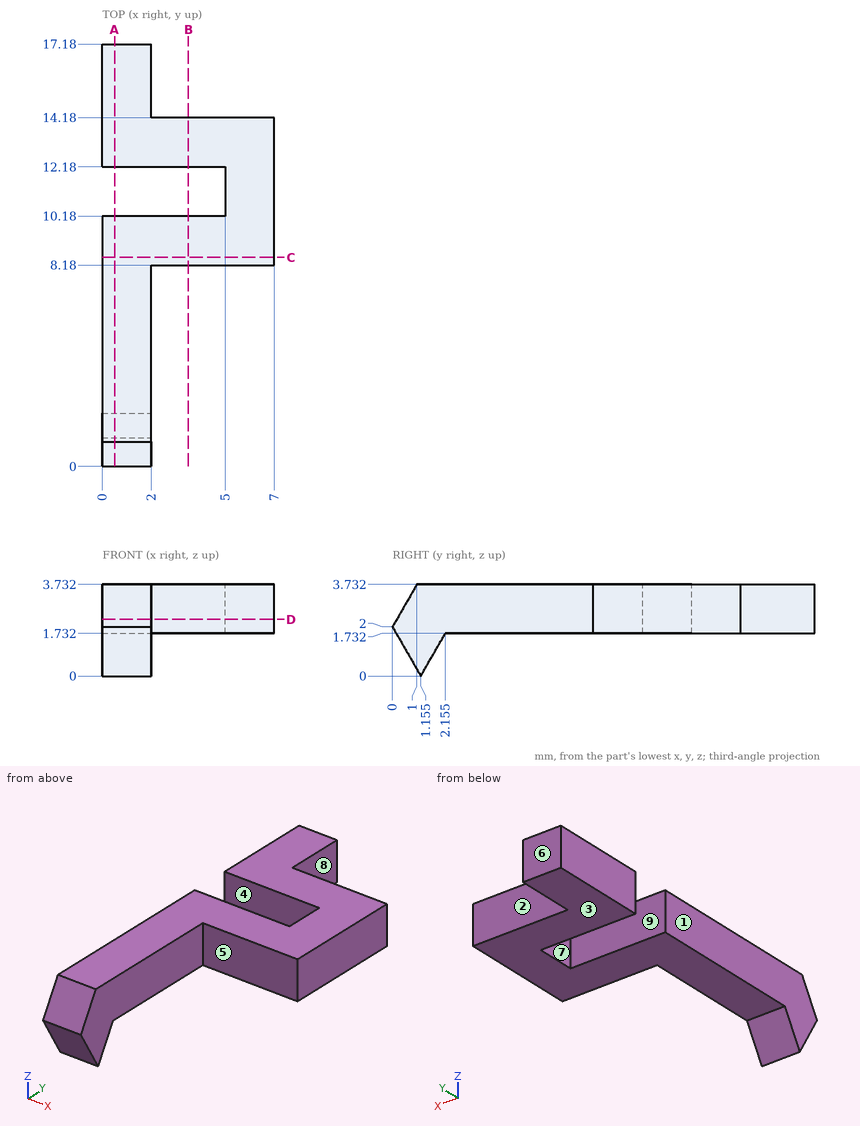
Geometry: see drawing. Coordinates: mm, zero at the bounding-box minimum. A direction names the side the tool comes from. Coordinates: 2 decimals unless noted, no trailing zeros. Order: outer loops, then holes, each group sorted by start corner. A loop starts at its lowest first (then second) coordinate and runs counter-clockwise, first axis right, second up. Notation, with made-up numbers: M -1,8 L 24,8 A22 ccw 24,16 Z; hole C 61.5,83.5 d4. An arc over 180 degrees is marked long. Write each question's results on one line, items separated by ' | '. Start each with the question number.
1) Access query for the marked faces 1, 2, 3, 4 and 5. Directions: +Z, -Z, +X, -X, +Y, -Y. A direction counts if a zero-diameter tool reaches every point of the face in a straight line with its end or side. Return the directions, or none.
2) Section query B-B (x = 3.5). Return the cut outline in (y, z).
3) Section query A-A (x = 0.5). Return the cut outline in (y, z) (1 decimal), plus the area to 3 significant figures.
4) Contact query for flat-ended pins moving along their axis: pin 1 Ø0.6 at (x, z) = (1.5, 2.5) entering from -Y (1 decimal); pin 2 Ø0.6 at (x, z) = (4.5, 2.5) entering from -Y; pin 3 Ø2 at (x, y) = (2, 7.5) entering from -Z. Output: stop coordinate, or through.
5) Section query D-D (z = 2.3). Return the cut outline in (x, y), plus the area to 3 significant figures.
6) Line query: line 1 (Y direction, x = 4.5, z = 2.65); line 2 (X direction, y = 12, z = 3.1); line 3 (Y direction, x = 5.75, z = 3.55). Output: solid intervals per line, ascending. Write a range as from..to.
7) Draft query along Y for the marked faces 6, 7, 8 and 9. Return one class per face: released by +Y, released by -Y, zero draft, split by the parting line, or undercut.
8) Section query C-C (y = 8.5). Return the cut outline in (x, z), plus the area to 3 significant figures.
Answers:
1) face 1: +Z, -Z, -X, +Y, -Y | face 2: +Z, -Z, +X, +Y | face 3: -Z, +X, -X, +Y | face 4: +Z, -Z, -X | face 5: +Z, -Z, +X, -Y
2) outline: M 8.18,1.73 L 10.18,1.73 L 10.18,3.73 L 8.18,3.73 Z; M 12.18,1.73 L 14.18,1.73 L 14.18,3.73 L 12.18,3.73 Z
3) outline: M 0,2 L 1.2,0 L 2.2,1.7 L 10.2,1.7 L 10.2,3.7 L 1,3.7 Z; M 12.2,1.7 L 17.2,1.7 L 17.2,3.7 L 12.2,3.7 Z | area: 31.2 mm^2
4) pin 1: stops at y = 0.1 | pin 2: stops at y = 8.18 | pin 3: stops at z = 1.73
5) outline: M 0,0.17 L 2,0.17 L 2,8.18 L 7,8.18 L 7,14.18 L 2,14.18 L 2,17.18 L 0,17.18 L 0,12.18 L 5,12.18 L 5,10.18 L 0,10.18 Z | area: 54.0 mm^2
6) line 1: y = 8.18..10.18, 12.18..14.18 | line 2: x = 5..7 | line 3: y = 8.18..14.18
7) face 6: released by +Y | face 7: undercut | face 8: zero draft | face 9: undercut
8) outline: M 0,1.73 L 7,1.73 L 7,3.73 L 0,3.73 Z | area: 14.0 mm^2
